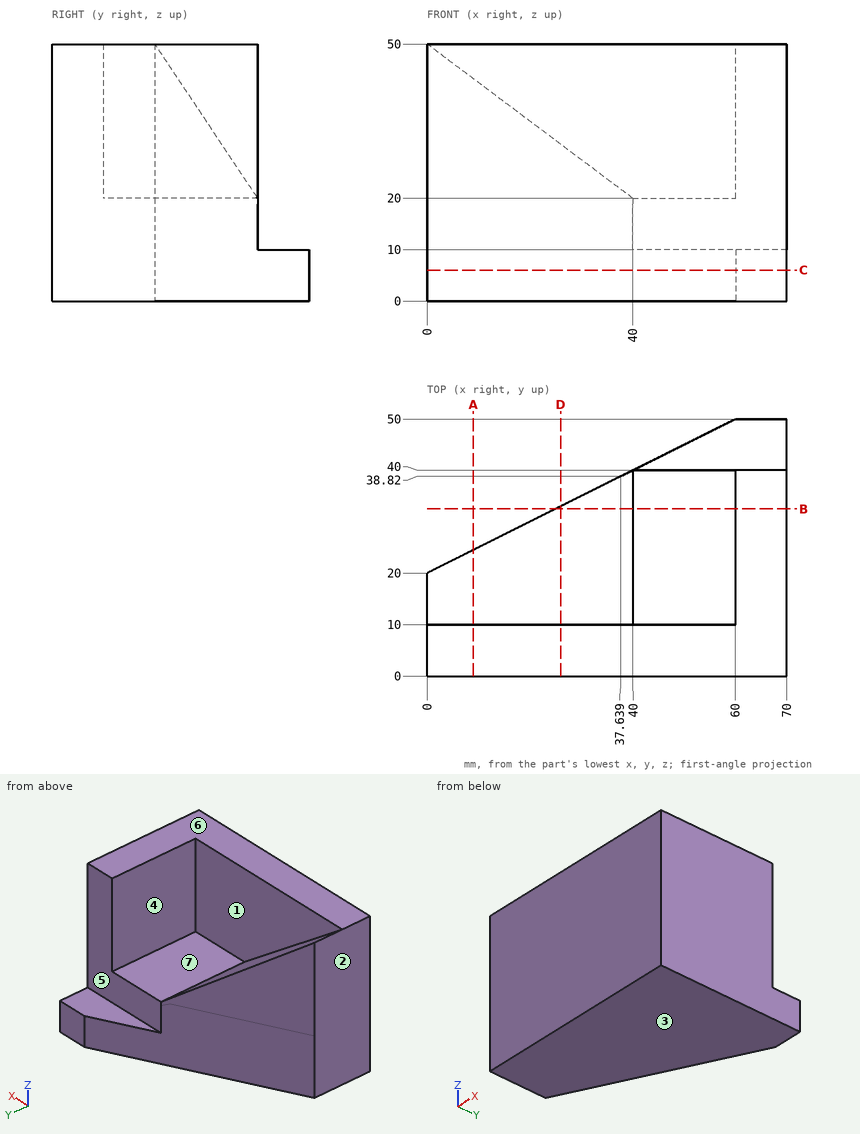
Input: dimensioned drawing with shaded views. Units: mm. Origin: part minimum x, y, z. A direction names the side the tool comes from. Coordinates: 2 decimals unless noted, no trailing zeros. Write each loop counter-clockwise with the first axis right and the second up, starting at its lowest first coordinate (ties: lowest second). Pieces come first, ordered by that corner, then holes. Notation, with made-up numbers: M 63,63.25 L 91,63.25 A16 ccw 91,73.25 Z; hole C 14.5,10.5 d4. An arc over 180 degrees is marked long. Answer as CSV lines item,"result". Start each with the question number.
Q1. Cut plane D-D on x = 26. Return the cut outline in (y, z).
Q2. Mould query, pull axis X, two halves, no side actions, for the marked faces 1, 2, 3 and 4. Classes: released by +X, released by -X, zero draft, split by the parting line, or undercut.
Q3. Cut plane B-B on y = 32.5. Return the cut outline in (x, z).
Q4. Cut plane A-A on x = 9. Return the cut outline in (y, z), then the cut area to 3 significant figures.
Q5. Line query: line 1 (Z direction, x = 49, y = 29.5); line 2 (Y direction, x = 24, z = 47.5); line 3 (X direction, y = 15, z = 21) (1 decimal). Output: solid intervals per line, ascending. Write a range as from..to.
Q6. Cut plane C-C on z = 6. Return the cut outline in (x, y), then the cut area to 3 significant figures.
Q7. Pin query (flat end, axial travel): P1, Ø2, axis at x = 62, z = 36, coming from the +Y side; P2, Ø8, axis at x = 23.5, z = 31, coming from the +Y side; P3, Ø1, axis at x = 34.5, z = 12.5, coming from the +Y side. Return the tip coordinate at first contact, or that it passes through.
Q8. Reachability of the marked faces 5, 6 and 7 from +Z, -Z, +X, -X, +Y, -Y: full face, straight path, thin tool, end or side. Return the list, or none.
Findings below:
1,outline,"M 0,0 L 33,0 L 33,30.5 L 10,30.5 L 10,50 L 0,50 Z"
2,face 1,"undercut"
2,face 2,"released by -X"
2,face 3,"zero draft"
2,face 4,"undercut"
3,outline,"M 25,0 L 70,0 L 70,50 L 60,50 L 60,20 L 40,20 L 25,31.25 Z"
4,outline,"M 0,0 L 24.5,0 L 24.5,43.25 L 10,43.25 L 10,50 L 0,50 Z"
4,area,"1,130 mm2"
5,line 1,"z = 0..20"
5,line 2,"y = 0..10"
5,line 3,"x = 0..38.7, 60..70"
6,outline,"M 0,0 L 70,0 L 70,50 L 60,50 L 0,20 Z"
6,area,"2,600 mm2"
7,P1,"stops at y = 40"
7,P2,"stops at y = 33.62"
7,P3,"stops at y = 37.5"
8,face 5,"+Z, +X, -X, +Y"
8,face 6,"+Z, +X, -X, +Y, -Y"
8,face 7,"+Z, +Y"
